Source: CAD feature listing. Evaluate the final solid. Frame: model axes, mm. A direction names the side the tool comes from. Give positions to 0.01 mm unless a question says otherwise; leave off trailing zeros. Order: outer loops, then holes, each group sorted by start corner. A loop starts at its lowest first (then second) coordinate and runs counter-clockwise, first axis right, second up. Notation, with made-up numbers: M -23,46 L 34,46 A13 cw 34,68 Z; hole C 65,26.5 d3. An arc over 180 degrees is marked long. Answer in a Markdown table with one row per item. Add a question column.
(1) Section query A-A, the plane x = 24. Return loops of the section in (y, z).
(2) Pin query (flat end, axial travel): P1, Ø6, axis at x = 84, z = -28, coming from the +Y side; P2, Ø8, axis at y = 50, z = 0, coming from the -X side; P3, Ø5, axis at x = 73, y = 180.5, coming from the -Z side; P4, Ø8, axis at x = 89.5, z = -87.5, coming from the +Y side. Return the tip coordinate at first contact, or that it passes through.
(3) Mould query, pull axis Y, two halves, no side actions, for faces 4 (the face through (193, -118, -111)), 5 (the face through (172.1, -110.161, -23.058)), 6 (the face through (95.149, 251.377, -55.821)). Classes: pulls with the +Y half, pulls with the -Y half, needs draft (parallel to the pull), parting line crosses it, or undercut.
(4) Material intervals for line 1 along Y through (x, z) = (60, 0); line 2 along Z through (x, y) = (145.5, 0); line 3 along X through (y, z) = (35, -49), sorted ascending.
(5) Section query C-C, the plane y = -223. Return loops of the section in (x, z).
(6) Section query B-B, the plane z = 198. Return loops of the section in (x, y).
(7) Set-up query: faces 1 (the face through (81.88, 153.755, -34.143)), 2 (the face through (188.07, 153.755, -34.143)), 3 (the face through (172.1, 105, -80.4)). Return all of +Z, -Z, +X, -X, +Y, -Y with unobstructed straight access to the full face (end or side cutting, diameter ignored); none if empty.
from build123d import *

# Parameters (mm, degrees)
F2_R     = 25
F3_DEPTH = 25
F4_R     = 5
F5_DEPTH = 66.501
F6_SIZE  = 5


with BuildPart() as f1:
    # F0 (on Front) → F1 (revolve)
    with BuildSketch(Plane.XZ):
        Polygon((193, 157.5), (193, 257.5), (0, 257.5), (0, 157.5), (161.5, 157.5), (161.5, 95.207259), (126.5, 75), (126.5, 28.5), (183, 28.5), (183, 157.5), align=None)
    revolve(axis=Axis((48.25, 0, 0), (1, 0, 0)))

    # F2 (on face) → F3 (cut)
    with BuildSketch(Plane(origin=(161.5, 0, 0), x_dir=(0, -1, 0), z_dir=(-1, 0, 0))):
        with Locations((7.845702, 130)):
            Circle(F2_R)
        with Locations((-58.205423, 116.506153)):
            Circle(F2_R)
        with Locations((-108.660452, 71.794577)):
            Circle(F2_R)
        with Locations((-130, 7.845702)):
            Circle(F2_R)
        with Locations((-116.506153, -58.205423)):
            Circle(F2_R)
        with Locations((-71.794577, -108.660452)):
            Circle(F2_R)
        with Locations((-7.845702, -130)):
            Circle(F2_R)
        with Locations((58.205423, -116.506153)):
            Circle(F2_R)
        with Locations((108.660452, -71.794577)):
            Circle(F2_R)
        with Locations((130, -7.845702)):
            Circle(F2_R)
        with Locations((116.506153, 58.205423)):
            Circle(F2_R)
        with Locations((71.794577, 108.660452)):
            Circle(F2_R)
    extrude(amount=-F3_DEPTH, mode=Mode.SUBTRACT)

    # F4 (on face) → F5 (cut, through all)
    with BuildSketch(Plane(origin=(126.5, 0, 0), x_dir=(0, -1, 0), z_dir=(-1, 0, 0))):
        with Locations((0, 50)):
            Circle(F4_R)
        with Locations((-50, 0)):
            Circle(F4_R)
        with Locations((0, -50)):
            Circle(F4_R)
        with Locations((50, 0)):
            Circle(F4_R)
    extrude(amount=-F5_DEPTH, mode=Mode.SUBTRACT)

    # F6
    f6_edges = [f1.edges().sort_by_distance(p)[0] for p in [
        (126.5, 0, -28.5),
    ]]
    chamfer(f6_edges, length=F6_SIZE)


solid = f1.part
Values follow:
| question | item | result |
|---|---|---|
| 1 | outline | C 0,0 d515; hole C 0,0 d315 |
| 2 | P1 | stops at y = 256.28 |
| 2 | P2 | passes through |
| 2 | P3 | stops at z = -186.07 |
| 2 | P4 | stops at y = 243.59 |
| 3 | face 4 | needs draft |
| 3 | face 5 | undercut |
| 3 | face 6 | parting line crosses it |
| 4 | line 1 | y = -257.5 to -157.5, 157.5 to 257.5 |
| 4 | line 2 | z = -257.5 to -157.5, -85.97 to -55, -45 to -28.5, 28.5 to 45, 55 to 85.97, 157.5 to 257.5 |
| 4 | line 3 | x = 126.5 to 183 |
| 5 | outline | M 0,-128.75 L 193,-128.75 L 193,128.75 L 0,128.75 Z |
| 6 | outline | M 0,-164.63 L 193,-164.63 L 193,164.63 L 0,164.63 Z |
| 7 | face 1 | -X |
| 7 | face 2 | +X |
| 7 | face 3 | +X, -X |
